```python
from build123d import *

# Parameters (mm, degrees)
SKETCH1_R           = 2.38125
BOSS_EXTRUDE1_DEPTH = 19.05
CHAMFER1_SIZE       = 0.508
SKETCH3_R           = 2.38125
BOSS_EXTRUDE2_DEPTH = 1.5875
SKETCH4_R           = 0.396875
CUT_EXTRUDE3_DEPTH  = 61.57513929


with BuildPart() as part:
    # Sketch1 → Boss-Extrude1 (new body)
    with BuildSketch(Plane.XY):
        with Locations(Location((0, 0, 0), (0, 0, 180))):
            Circle(SKETCH1_R)
    extrude(amount=BOSS_EXTRUDE1_DEPTH)

    # Chamfer1
    chamfer1_edges = [part.edges().sort_by_distance(p)[0] for p in [
        (2.38125, 0, 19.05),
    ]]
    chamfer(chamfer1_edges, length=CHAMFER1_SIZE)

    # Sketch3 → Boss-Extrude2 (add)
    with BuildSketch(Plane(origin=(0, 0, 0), x_dir=(-1, 0, 0), z_dir=(0, 0, -1))):
        with BuildLine():
            Line((0, 6.35), (50.8, 6.35))
            ThreePointArc((50.8, 6.35), (57.15, 0), (50.8, -6.35))
            Line((50.8, -6.35), (0, -6.35))
            ThreePointArc((0, -6.35), (-6.35, 0), (0, 6.35))
        make_face()
        with Locations((50.8, 0)):
            Circle(SKETCH3_R, mode=Mode.SUBTRACT)
    extrude(amount=BOSS_EXTRUDE2_DEPTH)

    # Sketch4 → Cut-Extrude3 (cut, through all)
    with BuildSketch(Plane.XY):
        with Locations((-12.7, 5.08)):
            Circle(SKETCH4_R)
    extrude(amount=-CUT_EXTRUDE3_DEPTH, mode=Mode.SUBTRACT)


solid = part.part
```
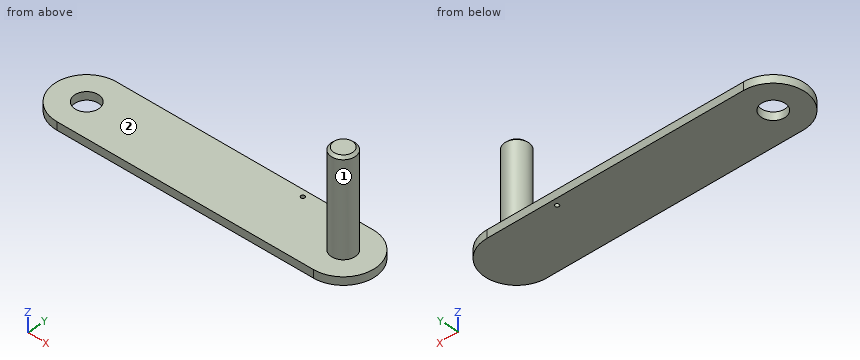
Here's how the part is built. I have some questions about the finished solid (model axes, mm). Face numbers are marked on the shaded views. Give positions to 0.01 mm unless a question says otherwise; leave off trailing zeros. Write each loop counter-clockwise with the first axis right and the second up, starting at its lowest first coordinate (ties: lowest second). Pieces come first, ordered by that corner, then holes.
(1) Imagine slicing it at A-A, the plane y = 0. Write out the boundary of the cut face in (x, z).
Output values:
outline: (-57.15, -1.59) - (-53.18, -1.59) - (-53.18, 0) - (-57.15, 0) - close; (-48.42, -1.59) - (6.35, -1.59) - (6.35, 0) - (2.38, 0) - (2.38, 18.54) - (1.87, 19.05) - (-1.87, 19.05) - (-2.38, 18.54) - (-2.38, 0) - (-48.42, 0) - close
(2) Imagine slicing it at B-B, the plane z = 9.75. Write out the boundary of the cut face in (x, y).
Output values:
outline: circle Ø4.76 at (0, 0)
(3) Imagine slicing it at C-C, the plane x = -23. Write out the boundary of the cut face in (y, z).
Output values:
outline: (-6.35, -1.59) - (6.35, -1.59) - (6.35, 0) - (-6.35, 0) - close
(4) If I drill on L1, parallel to Y at x = -50.8, z = -1; L2, parallel to Y at x = -12.7, z = -0.5; L3, parallel to Z at x = -24.5, y = 4.75, over which ranges is the centre line in solid material (lowest first)?
Output values:
L1: y = -6.35 to -2.38, 2.38 to 6.35
L2: y = -6.35 to 4.68, 5.48 to 6.35
L3: z = -1.59 to 0
(5) Will these pins go through, and if not, where does the flat tip stop? pin 1 (12 mm diameter, centred on x = -1, z = 14, fed in from +Y); pin 2 (4 mm diameter, centred on x = -38, y = -2.5, fed in from +Z); pin 3 (4 mm diameter, centred on x = -50.8, y = 0, fed in from -Z); pin 4 (1.5 mm diameter, centred on y = 0, z = 4.5, fed in from +X).
Output values:
pin 1: stops at y = 2.38
pin 2: stops at z = 0
pin 3: passes through
pin 4: stops at x = 2.38
(6) Imagine slicing it at D-D, the plane y = -4. Write out the boundary of the cut face in (x, z).
Output values:
outline: (-55.73, -1.59) - (4.93, -1.59) - (4.93, 0) - (-55.73, 0) - close
(7) Thinking about a two-plate mould opening in Y: for the marked faces 1 and 2, which applies, pulls with the +Y half, pulls with the -Y half, needs draft (parallel to the pull), parting line crosses it, or undercut?
Output values:
face 1: parting line crosses it
face 2: needs draft
